For this review, take the finished solid that the model builds, in its own axes (mm). A direction names the side the tool comes from. Give positions to 0.01 mm unless a question says otherwise; leave off trailing zeros. Loops run counter-clockwise (first coordinate to the right, second up) from the corner with the lowest first, then second, coordinate; pieces in that order, holes last. Notation, with made-up numbers: (35.5, 55) - (82.5, 55) arc R34 cw to (82.5, 94) - close; hole circle Ø1 at (37.25, 0.25). An arc over 180 degrees is marked (long way). Put each result on its own line as item: value.
Autodesk Inventor part; units mm, degrees
ref_plane "YZ Plane" through (0, 0, 0) normal (1, 0, 0) x (0, 1, 0)
ref_plane "XZ Plane" through (0, 0, 0) normal (0, 1, 0) x (-1, 0, 0)
ref_plane "XY Plane" through (0, 0, 0) normal (0, 0, 1) x (1, 0, 0)
sketch "スケッチ1" plane through (0, 0, 0) normal (0, 0, 1) x (1, 0, 0)
  line L0 (-24.25, -20) -> (24.25, -20) construction
  line L1 (24.25, -20) -> (24.25, 20)
  line L2 (24.25, 20) -> (-24.25, 20)
  line L3 (-24.25, 20) -> (-24.25, -20)
  line L4 (-24.25, -20) -> (24.25, 20) construction
  line L5 (24.25, -20) -> (-24.25, 20) construction
  circle A0 centre (-15.25, -17.5) radius 1.55
  circle A1 centre (20.25, -17.5) radius 1.55
  line L6 (-9.25, -15) -> (14.25, -15) construction
  line L7 (14.25, -15) -> (14.25, -20) construction
  line L8 (14.25, -20) -> (-9.25, -20) construction
  line L9 (-9.25, -20) -> (-9.25, -15) construction
  line L10 (-24.25, -20) -> (-15.25, -22)
  line L11 (-15.25, -22) -> (20.25, -22)
  line L12 (20.25, -22) -> (24.25, -20)
  line L13 (14.3, -14.95) -> (-9.3, -14.95)
  line L14 (-9.3, -14.95) -> (-9.3, -20.05)
  line L15 (-9.3, -20.05) -> (14.3, -20.05)
  line L16 (14.3, -20.05) -> (14.3, -14.95)
  circle A2 centre (-8.25, -14.95) radius 1.05
  circle A3 centre (-8.25, -20.05) radius 1.05
  circle A4 centre (13.25, -14.95) radius 1.05
  circle A5 centre (13.25, -20.05) radius 1.05
  circle A6 centre (-19.25, 15) radius 1.55
  line L17 (-21.8, 5.05) -> (-19.2, 5.05)
  line L18 (-19.2, 5.05) -> (-19.2, -15.05)
  line L19 (-19.2, -15.05) -> (-21.8, -15.05)
  line L20 (-21.8, -15.05) -> (-21.8, 5.05)
  line L21 (-19.25, 5) -> (-21.75, 5) construction
  line L22 (-21.75, 5) -> (-21.75, -15) construction
  line L23 (-21.75, -15) -> (-19.25, -15) construction
  line L24 (-19.25, -15) -> (-19.25, 5) construction
  line L25 (2.5, -14.95) -> (2.5, -20.05) construction
  circle A7 centre (-21.8, 4) radius 1.05
  circle A8 centre (-19.2, 4) radius 1.05
  circle A9 centre (-21.8, -14) radius 1.05
  circle A10 centre (-19.2, -14) radius 1.05
  line L26 (24.25, 6) -> (34.25, 6)
  line L27 (34.25, 6) -> (34.25, -6)
  line L28 (34.25, -6) -> (24.25, -6)
  line L29 (24.25, -6) -> (24.25, 6)
  circle A11 centre (29.25, 0) radius 1.55
  point P0 (0, 0)
  point P1 (-9.25, -17.5)
  dimension "d10" = 2.1
  dimension "d26" = 2.1
  dimension "d0" = 5
  dimension "d3" = 3.1
  dimension "d4" = 35.5
  dimension "d5" = 2
  dimension "d7" = 40
  dimension "d8" = 23.5
  dimension "d9" = 0.05
  dimension "d11" = 3.1
  dimension "d12" = 5
  dimension "d13" = 5
  dimension "d14" = 0.05
  dimension "d15" = 17.75
  dimension "d16" = 48.5
  dimension "d17" = 4
  dimension "d20" = 2.5
  dimension "d21" = 2.5
  dimension "d22" = 5
  dimension "d23" = 15
  dimension "d27" = 25
  dimension "d57" = 10
  dimension "d58" = 3.1
  dimension "d59" = 5
  dimension "d60" = 6
  dimension "d61" = 12
  dimension "d62" = 20
extrude "押し出し1" add sketch "スケッチ1" along normal blind 5
sketch "スケッチ2" plane through (0, 0, 0) normal (0, 0, -1) x (-1, 0, 0)
  line L0 (-14.3, -20.05) -> (-14.3, -14.95)
  line L1 (-12.2, -14.95) -> (7.2, -14.95)
  line L2 (24.25, 20) -> (-24.25, 20)
  line L3 (-24.25, 20) -> (-24.25, -20)
  line L4 (21.8, -15.05) -> (19.2, -15.05)
  line L5 (19.2, -12.95) -> (19.2, 2.95)
  line L6 (19.2, 5.05) -> (21.8, 5.05)
  line L7 (-20.25, 16) -> (16.25, 16)
  line L8 (16.25, 16) -> (16.25, -11)
  line L9 (16.25, -11) -> (-20.25, -11)
  line L10 (-20.25, -11) -> (-20.25, -5.9161)
  line L11 (-20.25, 16) -> (-20.25, 5.9161)
  line L12 (19.25, 5.05) -> (19.25, -15.05) construction
  line L13 (19.2, -15.05) -> (21.8, -15.05)
  line L14 (-14.3, -15) -> (9.3, -15) construction
  line L15 (9.3, -20.05) -> (9.3, -14.95)
  line L16 (-20.25, 5.9161) -> (-20.25, -5.9161)
  point P0 (0, 0)
  dimension "d29" = 4
  dimension "d30" = 4
  dimension "d31" = 0.05
  dimension "d32" = 3
  dimension "d33" = 0.05
  dimension "d34" = 4
sketch "スケッチ3" plane through (0, 0, 0) normal (0, 0, -1) x (-1, 0, 0)
  circle A0 centre (15.25, -17.5) radius 1.55
  circle A1 centre (15.25, -17.5) radius 3
  circle A2 centre (19.25, 15) radius 1.55
  circle A3 centre (19.25, 15) radius 3
  circle A4 centre (-20.25, -17.5) radius 3
  point P0 (0, 0)
  dimension "d38" = 6
  dimension "d39" = 6
  dimension "d40" = 6
extrude "押し出し3" cut sketch "スケッチ3" against normal blind 3.5 contours A1 | A4
extrude "押し出し5" cut sketch "スケッチ2" against normal blind 3
fillet "フィレット4" radius 2 4 edges at (20.25, -11, 1.5) (20.25, 16, 1.5) (-16.25, 16, 1.5) (-16.25, -11, 1.5)
fillet "フィレット5" radius 2 4 edges at (24.25, -6, 2.5) (34.25, -6, 2.5) (34.25, 6, 2.5) (24.25, 6, 2.5)
equation "\"d13\" = d12"
equation "\"d15\" = 0.5 * d4"
equation "\"d59\" = 0.5 * d57"
properties part number "コックピット_サブフレーム_1_5" material "アセタール樹脂、黒"
1) Take a section at C-C on x = -1.5. State the section outline as (y, z) points, and give its area (4 significant figures).
Geometry check:
outline: (-22, 0) - (-20.05, 0) - (-20.05, 5) - (-22, 5) - close; (-14.95, 0) - (-11, 0) - (-11, 3) - (16, 3) - (16, 0) - (20, 0) - (20, 5) - (-14.95, 5) - close
area: 103.5 mm²
2) Draft analysis for pull direction Y (two halves, no side actions). For faces 1 (the face through (24.25, -14, 2)), 2 (the face through (29, -6, 2)), 3 (the face through (-22.85, 3.98, 2.46)), state which applies: pulls with the +Y half, pulls with the -Y half, needs draft (parallel to the pull), parting line crosses it, or undercut.
Geometry check:
face 1: needs draft
face 2: pulls with the -Y half
face 3: undercut
3) For faces 4 (the face through (-16.25, 3, 1)), 5 (the face through (-21, 5.05, 2)), 6 (the face through (24.85, -6.57, 2.54)), list the 3-axis set-ups (+Z, -Z, +X, -X, +Y, -Y) from which the entire face can be reached by the end or side of a thin tool; tool diameter is ignored.
Geometry check:
face 4: -Z
face 5: +Z, -Z
face 6: +Z, -Z, +X, -Y
4) Insertion check: pin 1 Ø3 at (x, z) = (-21, 2.5) entering from -Y; pin 2 Ø3.5 at (x, y) = (20.25, -17.5) entering from -Z; pin 3 Ø1 at (x, y) = (12.5, 15) entering from -Z. Each pin has a flat end and moves straight along its axis. Give the tip position at first contact, or say it passes through.
Geometry check:
pin 1: stops at y = -21.06
pin 2: stops at z = 3.5
pin 3: stops at z = 3
5) Take a section at A-A on z = 4.1. State how many separate pieces and enclosed holes the cut face has, and give its area (3 significant figures).
Geometry check:
separate pieces: 1
enclosed holes: 6
area: 1,930 mm²
6) Take a section at B-B on x = 13.25. State the section outline as (y, z) points, and give its area (3 significant figures).
Geometry check:
outline: (-22, 0) - (-21.1, 0) - (-21.1, 5) - (-22, 5) - close; (-13.9, 0) - (-11, 0) - (-11, 3) - (16, 3) - (16, 0) - (20, 0) - (20, 5) - (-13.9, 5) - close
area: 93.0 mm²
7) Wall thickness on line 1 (X direction, y = -2, z = 1.9); line 2 (Y direction, x = 11, z = 1.2); line 3 (Y direction, x = 29.25, z = 2.95): over which ranges is each line inside the solid? List them lowest first.
Geometry check:
line 1: x = -24.25 to -21.8, -19.2 to -16.25, 20.25 to 34.25
line 2: y = -22 to -20.05, -14.95 to -11, 16 to 20
line 3: y = -6 to -1.55, 1.55 to 6
